Check sheet for the modelled part. Datum: model origin and axes. Units: mm. A direction names the side the tool comes from. Give positions to 0.01 mm unless a question says otherwise; leave off trailing zeros. Loops run counter-clockwise (first coordinate to the right, second up) from the corner with the lowest first, then second, coordinate; pieces in that order, holes last. Notation, with made-up numbers: (-21, 70) -> (-3, 70) arc R19 ccw to (-3, 92) -> close; hole circle Ø1 at (-35, 51.25). An arc over 180 degrees is marked (long way). Answer as CSV lines item,"result". Start each with the question number.
(1) Access from +Z, -Z, +X, -X, +Y, -Y to the whole of each face (thin tool, end or side, straight path). Record for faces 4 (the face through (0, 0, 9)), 5 (the face through (0, 0.5, 1)).
(2) Section check D-D on z = 11.25. Enter the section's corners in (x, y), plus the area to 3 significant figures.
(3) Material ranges on line 1 (Z direction, x = 0.05, y = 0.15); line 2 (Z direction, x = -1, y = 0.8); line 3 (X direction, y = 0.3, z = 5.25), recorded low to high. Write a range as from..to.
(4) Section check C-C on y = 0.5. Enter the section's corners in (x, z), plus the area to 3 significant figures.
(5) Gauge pin test, flat end, axial feed: pin 1 Ø0.6 at (y, z) = (0.5, 5) entering from -X. Record the tip position at first contact, or that the pin passes through.
(6) Release check for a two-part mould opening along X. For faces 1 (the face through (0, 0.4, 0)), 2 (the face through (0, 1, 9)), 3 (the face through (0, 0.5, 7.5)) record: pulls with the +X half, pulls with the -X half, needs draft (parallel to the pull), parting line crosses it, or undercut.
(7) Section check B-B on z = 2.5. Enter the section's corners in (x, y).
(8) Section check A-A on x = 0. Enter the section's corners in (y, z).
from build123d import *

# Parameters (mm, degrees)
BOSS_EXTRUDE1_DEPTH = 14.5
CUT_EXTRUDE1_DEPTH  = 15.773286703


with BuildPart() as part:
    # Sketch1 → Boss-Extrude1 (new body)
    with BuildSketch(Plane.XY):
        with BuildLine():
            Line((-2.645751311, 0), (2.645751311, 0))
            ThreePointArc((2.645751311, 0), (0, 1), (-2.645751311, 0))
        make_face()
    extrude(amount=BOSS_EXTRUDE1_DEPTH)

    # Sketch2 → Cut-Extrude1 (cut, through all)
    with BuildSketch(Plane.XZ):
        with BuildLine():
            Line((-1.25, 2.25), (-1.25, 6.25))
            ThreePointArc((-1.25, 6.25), (0, 7.5), (1.25, 6.25))
            Line((1.25, 6.25), (1.25, 2.25))
            ThreePointArc((1.25, 2.25), (0, 1), (-1.25, 2.25))
        make_face()
    extrude(amount=-CUT_EXTRUDE1_DEPTH, mode=Mode.SUBTRACT)


solid = part.part
Working result:
1,face 4,"+Z, -Z, +X, -X, -Y"
1,face 5,"+Y, -Y"
2,outline,"(-2.65, 0) -> (2.65, 0) arc R4 ccw to start"
2,area,"3.63 mm^2"
3,line 1,"z = 0..1, 7.5..14.5"
3,line 2,"z = 0..1.5, 7..14.5"
3,line 3,"x = -2.26..-1.25, 1.25..2.26"
4,outline,"(-1.94, 0) -> (1.94, 0) -> (1.94, 14.5) -> (-1.94, 14.5) -> close; hole (-1.25, 2.25) arc R1.25 ccw to (1.25, 2.25) -> (1.25, 6.25) arc R1.25 ccw to (-1.25, 6.25) -> close"
4,area,"41.2 mm^2"
5,pin 1,"stops at x = -2.4"
6,face 1,"needs draft"
6,face 2,"parting line crosses it"
6,face 3,"undercut"
7,outline,"(-2.65, 0) -> (-1.25, 0) -> (-1.25, 0.8) arc R4 ccw to start; (1.25, 0) -> (2.65, 0) arc R4 ccw to (1.25, 0.8) -> close"
8,outline,"(0, 0) -> (1, 0) -> (1, 1) -> (0, 1) -> close; (0, 7.5) -> (1, 7.5) -> (1, 14.5) -> (0, 14.5) -> close"
